Autodesk Inventor part; units mm, degrees
ref_plane "YZ Plane" through (0, 0, 0) normal (1, 0, 0) x (0, 1, 0)
ref_plane "XZ Plane" through (0, 0, 0) normal (0, 1, 0) x (-1, 0, 0)
ref_plane "XY Plane" through (0, 0, 0) normal (0, 0, 1) x (1, 0, 0)
sketch "Sketch1" plane through (0, 0, 0) normal (0, 0, 1) x (1, 0, 0)
  line L0 (0, -23) -> (0, 23)
  line L1 (0, -23) -> (-22, 0)
  line L2 (-22, 0) -> (0, 23)
  point P0 (0, 0)
  point P1 (0, 0)
  point P2 (0, 0)
  dimension "d1" = 46
  dimension "d9" = 22
extrude "Plate1" add sketch "Sketch1" along normal blind 2
fillet "Corner Round2" radius 1 3 edges at (0, -23, 1) (-22, 0, 1) (0, 23, 1)
equation "\"d2\" = Thickness"
equation "\"BendReliefWidth\" = Thickness"
equation "\"BendReliefDepth\" = 0.5 * Thickness"
equation "\"CornerReliefSize\" = 4 * Thickness"
equation "\"MinimumRemnant\" = 2 * Thickness"
equation "\"TransitionRadius\" = BendRadius"
equation "\"JacobiRadiusSize\" = BendRadius"
equation "\"GapSize\" = Thickness"
properties part number "MNT-CDF-605 CAP" material "Stainless Steel"
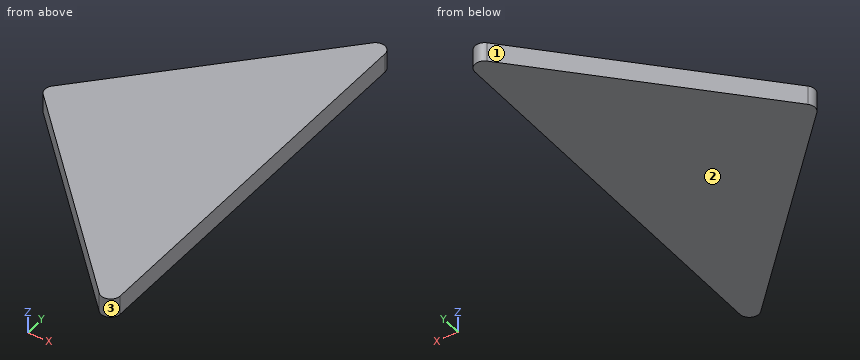
Design review of the part built by this model. Coordinates are the model's own, in mm. Face numbers are marked on the shaded views. Coordinates: 2 decimals unless noted, no trailing zeros. Order: outer loops, then holes, each group sorted by start corner. A loop starts at its lowest first (then second) coordinate and runs counter-clockwise, first axis right, second up. Notation, with made-up numbers: (-0.5, -7.5) -> (21.5, -7.5) arc R20 ccw to (21.5, 7.5) -> close; hole circle Ø9 at (8, 16). An arc over 180 degrees is marked (long way). Use one line per item in the form item = value. Start each with the question number.
(1) Add section C-C on y = 7.5. State the section outline as (x, z) points.
(2) For probe 1 along X at (y, z) = (-12.5, 0.3); probe 2 along Y at (x, z) = (-19.75, 0.35); probe 3 along X at (y, z) = (15, 0.1), list the stretches that pass through material, from the lowest coordinate up.
(3) The part is to be moulded in two halves that separate along X. For the marked faces 1, 2 and 3, say which applies: +X half, -X half, draft (parallel to the pull), parting line (faces both ways), or undercut.
(4) Insertion check: pin 1 (5 mm diameter, centred on x = -12, y = 14.5, fed in from -Z). The pin has a flat end and moves straight along its axis. Give the tip position at first contact, or say it passes through.
(5) Add section A-A on z = 0.35. State the section outline as (x, y) points.
(6) Add section B-B on x = -16.5. State the section outline as (y, z) points, plus the area to 3 significant figures.
Answer block:
q1.outline = (-14.83, 0) -> (0, 0) -> (0, 2) -> (-14.83, 2) -> close
q2.probe_1 = -10.04 to 0
q2.probe_2 = -2.35 to 2.35
q2.probe_3 = -7.65 to 0
q3.face_1 = -X half
q3.face_2 = draft
q3.face_3 = parting line
q4.pin_1 = through
q5.outline = (-21.34, -0.69) -> (-1.72, -21.2) arc R1 ccw to (0, -20.51) -> (0, 20.51) arc R1 ccw to (-1.72, 21.2) -> (-21.34, 0.69) arc R1 ccw to start
q6.outline = (-5.75, 0) -> (5.75, 0) -> (5.75, 2) -> (-5.75, 2) -> close
q6.area = 23.0 mm²
